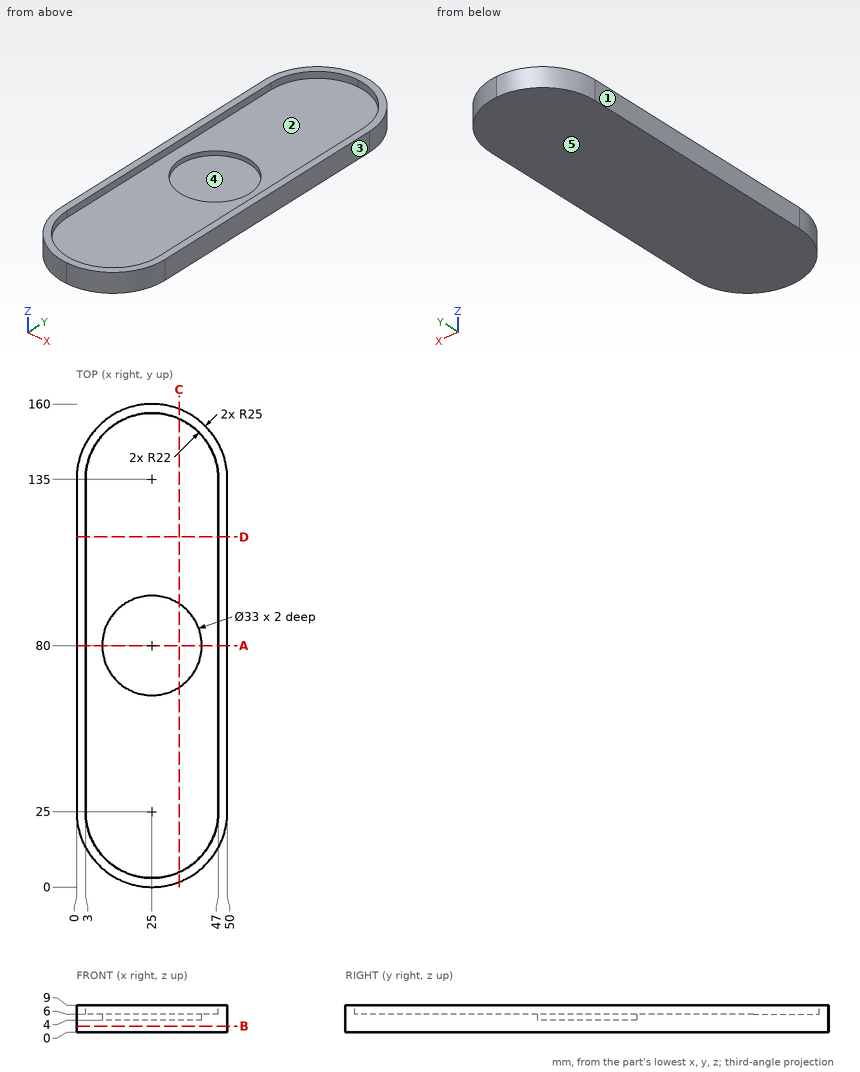
Could you check a few things on this drawing? It's one solid part, dimensions in mm from its lowest x, y, z. A direction names the side the tool comes from. Give positions to 0.01 mm unless a question says otherwise; leave off trailing zeros. Order: outer loops, then holes, each group sorted by start corner. A loop starts at its lowest first (then second) coordinate and runs counter-clockwise, first axis right, second up. Notation, with made-up numbers: (54.25, 6.5) -> (108.25, 6.5) arc R22 cw to (108.25, 30.5) -> close; hole circle Ø1 at (78.25, 54.5). An arc over 180 degrees is marked (long way). Use CSV: the item, a comma, the result in double quotes. Start each with the question number.
Item 1: Thinking about a two-plate mould opening in X: for the marked faces 1, 2 and 3, which applies, pulls with the +X half, pulls with the -X half, needs draft (parallel to the pull), parting line crosses it, or undercut?
Item 2: Suppose I cut it at C-C (x = 34). List the corners of the cut face in (y, z) for me.
Item 3: On a 3-axis mill with a long thin cutter (end or side, diameter ignored), from which of +Z, -Z, +X, -X, +Y, -Y can I reach the whole of each face in a straight line? I mean the marked faces 4 and 5. Say none if no direction works.
Item 4: Suppose I cut it at A-A (y = 80). List the corners of the cut face in (x, z) for me.
Item 5: I'm going to push flat-ended pins straight in: P1, Ø10, axis at x = 31.5, y = 64, coming from the +Z side; P2, Ø5, axis at x = 35, z = 1.5, coming from the -Y side; P3, Ø10, axis at x = 23, y = 73, coming from the +Z side. Where does each tip first touch, or does it pass through?
Item 6: If I drill on probe 1 along Z at (x, y) = (4, 122.5); probe 2 along X at (y, z) = (40.5, 7.5); probe 3 along Z at (x, y) = (25.5, 91), over which ranges is the centre line in solid material (lowest first)? Write a range as [from, to].
Item 7: Suppose I cut it at B-B (z = 2). List the corners of the cut face in (x, y) for me, and give its area (3 significant figures).
Item 8: Suppose I cut it at D-D (y = 116). List the corners of the cut face in (x, z) for me, and give its area (3 significant figures).
Answer block:
1,face 1,"pulls with the -X half"
1,face 2,"undercut"
1,face 3,"pulls with the +X half"
2,outline,"(1.68, 0) -> (158.32, 0) -> (158.32, 9) -> (155.07, 9) -> (155.07, 6) -> (93.83, 6) -> (93.83, 4) -> (66.17, 4) -> (66.17, 6) -> (4.93, 6) -> (4.93, 9) -> (1.68, 9) -> close"
3,face 4,"+Z"
3,face 5,"-Z, +X, -X, +Y, -Y"
4,outline,"(0, 0) -> (50, 0) -> (50, 9) -> (47, 9) -> (47, 6) -> (41.5, 6) -> (41.5, 4) -> (8.5, 4) -> (8.5, 6) -> (3, 6) -> (3, 9) -> (0, 9) -> close"
5,P1,"stops at z = 6"
5,P2,"stops at y = 1.15"
5,P3,"stops at z = 4"
6,probe 1,"z = [0, 6]"
6,probe 2,"x = [0, 3], [47, 50]"
6,probe 3,"z = [0, 4]"
7,outline,"(0, 25) arc R25 ccw to (25, 0) arc R25 ccw to (50, 25) -> (50, 135) arc R25 ccw to (25, 160) arc R25 ccw to (0, 135) -> close"
7,area,"7,460 mm^2"
8,outline,"(0, 0) -> (50, 0) -> (50, 9) -> (47, 9) -> (47, 6) -> (3, 6) -> (3, 9) -> (0, 9) -> close"
8,area,"318 mm^2"
